```python
from build123d import *

# Parameters (mm, degrees)
F0_R     = 55.8806252639
F1_DEPTH = 12.7


with BuildPart() as f1:
    # F0 (on Top) → F1 (new body)
    with BuildSketch(Plane.XY):
        Circle(F0_R)
        with BuildLine():
            add(Edge.make_bspline(
                [(-8.8274130972, -11.1133217732), (-11.8591704488, -9.6938284468), (-14.8909278004, -9.6938284468)],
                knots=[0, 0, 0, 1, 1, 1], degree=2))
            add(Edge.make_bspline(
                [(-14.8909278004, -9.6938284468), (-19.2896046515, -9.6938284468), (-21.8365144883, -12.6233589127)],
                knots=[0, 0, 0, 1, 1, 1], degree=2))
            add(Edge.make_bspline(
                [(-21.8365144883, -12.6233589127), (-24.3834243251, -15.5528893786), (-24.3834243251, -20.6467090522)],
                knots=[0, 0, 0, 1, 1, 1], degree=2))
            add(Edge.make_bspline(
                [(-24.3834243251, -20.6467090522), (-24.3834243251, -25.8807255975), (-21.9270583013, -28.7401576276)],
                knots=[0, 0, 0, 1, 1, 1], degree=2))
            add(Edge.make_bspline(
                [(-21.9270583013, -28.7401576276), (-19.4706922775, -31.5995896577), (-14.9259770183, -31.5995896577)],
                knots=[0, 0, 0, 1, 1, 1], degree=2))
            add(Edge.make_bspline(
                [(-14.9259770183, -31.5995896577), (-12.133722656, -31.5995896577), (-8.55286089, -30.5948454101)],
                knots=[0, 0, 0, 1, 1, 1], degree=2))
            Line((-8.55286089, -30.5948454101), (-8.55286089, -33.3111598003))
            add(Edge.make_bspline(
                [(-8.55286089, -33.3111598003), (-11.3275906434, -34.3567948021), (-15.3991414605, -34.3567948021)],
                knots=[0, 0, 0, 1, 1, 1], degree=2))
            add(Edge.make_bspline(
                [(-15.3991414605, -34.3567948021), (-21.2932516103, -34.3567948021), (-24.4973342834, -30.7759330361)],
                knots=[0, 0, 0, 1, 1, 1], degree=2))
            add(Edge.make_bspline(
                [(-24.4973342834, -30.7759330361), (-27.7014169565, -27.1950712702), (-27.7014169565, -20.605818298)],
                knots=[0, 0, 0, 1, 1, 1], degree=2))
            add(Edge.make_bspline(
                [(-27.7014169565, -20.605818298), (-27.7014169565, -16.481693654), (-26.1592513673, -13.3798378665)],
                knots=[0, 0, 0, 1, 1, 1], degree=2))
            add(Edge.make_bspline(
                [(-26.1592513673, -13.3798378665), (-24.617085778, -10.2779820791), (-21.705079921, -8.5985403862)],
                knots=[0, 0, 0, 1, 1, 1], degree=2))
            add(Edge.make_bspline(
                [(-21.705079921, -8.5985403862), (-18.7930740641, -6.9190986934), (-14.8500370461, -6.9190986934)],
                knots=[0, 0, 0, 1, 1, 1], degree=2))
            add(Edge.make_bspline(
                [(-14.8500370461, -6.9190986934), (-10.6558139663, -6.9190986934), (-7.5130674245, -8.44958121)],
                knots=[0, 0, 0, 1, 1, 1], degree=2))
            Line((-7.5130674245, -8.44958121), (-8.8274130972, -11.1133217732))
        make_face(mode=Mode.SUBTRACT)
        Polygon((-2.8433452334, 4.6599686343), (2.6139786014, 4.792393521), (5.4573238349, 0.1324248867), (2.8433452334, -4.6599686343), (-2.6139786014, -4.792393521), (-5.4573238349, -0.1324248867), align=None, mode=Mode.SUBTRACT)
        with BuildLine():
            add(Edge.make_bspline(
                [(13.118225471, -17.7074033137), (15.3172801058, -17.2663672866), (17.5040837399, -17.2663672866)],
                knots=[0, 0, 0, 1, 1, 1], degree=2))
            add(Edge.make_bspline(
                [(17.5040837399, -17.2663672866), (21.926695011, -17.2663672866), (24.4626521665, -19.4592964211)],
                knots=[0, 0, 0, 1, 1, 1], degree=2))
            add(Edge.make_bspline(
                [(24.4626521665, -19.4592964211), (26.998609322, -21.6522255555), (26.998609322, -25.4622867892)],
                knots=[0, 0, 0, 1, 1, 1], degree=2))
            add(Edge.make_bspline(
                [(26.998609322, -25.4622867892), (26.998609322, -29.8052665554), (24.2329459024, -32.276905957)],
                knots=[0, 0, 0, 1, 1, 1], degree=2))
            add(Edge.make_bspline(
                [(24.2329459024, -32.276905957), (21.4672824829, -34.7485453585), (16.6036351847, -34.7485453585)],
                knots=[0, 0, 0, 1, 1, 1], degree=2))
            add(Edge.make_bspline(
                [(16.6036351847, -34.7485453585), (11.8747488947, -34.7485453585), (9.3877957422, -33.2355467658)],
                knots=[0, 0, 0, 1, 1, 1], degree=2))
            Line((9.3877957422, -33.2355467658), (9.3877957422, -30.172796578))
            add(Edge.make_bspline(
                [(9.3877957422, -30.172796578), (10.7231548241, -31.0303666306), (12.7139424462, -31.5204066606)],
                knots=[0, 0, 0, 1, 1, 1], degree=2))
            add(Edge.make_bspline(
                [(12.7139424462, -31.5204066606), (14.7047300682, -32.0104466906), (16.6403881869, -32.0104466906)],
                knots=[0, 0, 0, 1, 1, 1], degree=2))
            add(Edge.make_bspline(
                [(16.6403881869, -32.0104466906), (20.0094133935, -32.0104466906), (21.8746282578, -30.4208793432)],
                knots=[0, 0, 0, 1, 1, 1], degree=2))
            add(Edge.make_bspline(
                [(21.8746282578, -30.4208793432), (23.7398431222, -28.8313119957), (23.7398431222, -25.8236913113)],
                knots=[0, 0, 0, 1, 1, 1], degree=2))
            add(Edge.make_bspline(
                [(23.7398431222, -25.8236913113), (23.7398431222, -19.9677129523), (16.5668821824, -19.9677129523)],
                knots=[0, 0, 0, 1, 1, 1], degree=2))
            add(Edge.make_bspline(
                [(16.5668821824, -19.9677129523), (14.7476085709, -19.9677129523), (11.7032348842, -20.5251334864)],
                knots=[0, 0, 0, 1, 1, 1], degree=2))
            Line((11.7032348842, -20.5251334864), (10.0554752832, -19.4715474218))
            Line((10.0554752832, -19.4715474218), (11.1090613478, -6.3752276189))
            Line((11.1090613478, -6.3752276189), (25.0261982011, -6.3752276189))
            Line((25.0261982011, -6.3752276189), (25.0261982011, -9.3032167984))
            Line((25.0261982011, -9.3032167984), (13.8287835145, -9.3032167984))
            Line((13.8287835145, -9.3032167984), (13.118225471, -17.7074033137))
        make_face(mode=Mode.SUBTRACT)
        Polygon((-8.8821777954, 5.6402049959), (-11.8495973103, 5.6402049959), (-14.9195276811, 13.4795878234), (-24.7983370116, 13.4795878234), (-27.830500225, 5.6402049959), (-30.7331760414, 5.6402049959), (-20.9892494161, 30.3938790583), (-18.5775466468, 30.3938790583), align=None, mode=Mode.SUBTRACT)
        with BuildLine():
            Line((18.6679722386, 13.2637759067), (24.385376429, 29.3535589635))
            Line((24.385376429, 29.3535589635), (27.5124241231, 29.3535589635))
            Line((27.5124241231, 29.3535589635), (18.4982025739, 4.3317009695))
            Line((18.4982025739, 4.3317009695), (15.6230711564, 4.3317009695))
            Line((15.6230711564, 4.3317009695), (6.6526611336, 29.3535589635))
            Line((6.6526611336, 29.3535589635), (9.7358973013, 29.3535589635))
            Line((9.7358973013, 29.3535589635), (15.4861601365, 13.1651999724))
            add(Edge.make_bspline(
                [(15.4861601365, 13.1651999724), (16.4773959204, 10.3722151668), (17.0578986448, 7.7380471442)],
                knots=[0, 0, 0, 1, 1, 1], degree=2))
            add(Edge.make_bspline(
                [(17.0578986448, 7.7380471442), (17.6767364546, 10.5091261867), (18.6679722386, 13.2637759067)],
                knots=[0, 0, 0, 1, 1, 1], degree=2))
        make_face(mode=Mode.SUBTRACT)
    extrude(amount=F1_DEPTH)


solid = f1.part
```
Geometry: final body of the model. Coordinates: model frame, mm. Round coordinates to 2 decimals unless told otherwise and drop trailing zeros. Order: outer loops, then holes, each group sorted by start corner. A loop starts at its lowest first (then second) coordinate and runs counter-clockwise, first axis right, second up. Notation, with made-up numbers: (-4.75, -30.5) -> (54.25, -30.5) arc R16 cw to (54.25, -3.5) -> close; hole circle Ø4 at (37, -6.75). An arc over 180 degrees is marked (long way). Use one line per item in the form item = value. Start each with the question number.
1. Pin query (flat end, axial travel): pin 1 Ø6.5 at (x, z) = (17, 9) entering from -Y; pin 2 Ø2.5 at (x, z) = (7.5, 7) entering from -Y; pin 3 Ø3 at (y, z) = (-32, 3) entering from -X. Return the tip coordinate at first contact, or that it passes through.
2. Cut plane C-C (y = 16). Return the cut outline in (x, z), then the cut area to 3 significant figures.
3. Cut plane D-D (x = -13.5). Count the separate pieces of the cut face and the enclosed holes in it, then the cut area to 3 significant figures.
4. Draft query along X for faces 1 (the face through (-44.345, -34.002, 6.261)), 2 (the face through (9.388, -32, 6)), 3 (the face through (12, 1, 0)). Return one class per face: pulls with the +X half, pulls with the -X half, needs draft (parallel to the pull), parting line crosses it, or undercut.
5. Cut plane A-A (y = 2.5). Return the cut outline in (x, z), then the cut area to 3 significant figures.
6. Line query: probe 1 along X at (y, z) = (19, 3.25); probe 2 along X at (y, z) = (11, 8); probe 3 along X at (y, z) = (-32.5, 3.75). Output: solid intervals per line, ascending.
7. Cut plane B-B (x = 0). Return the cut outline in (y, z), then the cut area to 3 significant figures.
Solution:
q1.pin_1 = -54.16
q1.pin_2 = -55.53
q1.pin_3 = -46.82
q2.outline = (-53.54, 0) -> (-26.66, 0) -> (-26.66, 12.7) -> (-53.54, 12.7) -> close; (-12.94, 0) -> (11.44, 0) -> (11.44, 12.7) -> (-12.94, 12.7) -> close; (14.48, 0) -> (19.64, 0) -> (19.64, 12.7) -> (14.48, 12.7) -> close; (22.7, 0) -> (53.54, 0) -> (53.54, 12.7) -> (22.7, 12.7) -> close
q2.area = 1,110 mm^2
q3.separate_pieces = 4
q3.enclosed_holes = 0
q3.area = 1,210 mm^2
q4.face_1 = parting line crosses it
q4.face_2 = undercut
q4.face_3 = needs draft
q5.outline = (-55.82, 0) -> (-4.02, 0) -> (-4.02, 12.7) -> (-55.82, 12.7) -> close; (4.01, 0) -> (55.82, 0) -> (55.82, 12.7) -> (4.01, 12.7) -> close
q5.area = 1,320 mm^2
q6.probe_1 = -52.55 to -25.47, -14.11 to 10.36, 13.41 to 20.71, 23.78 to 52.55
q6.probe_2 = -54.79 to -28.62, -25.76 to -13.95, -10.98 to 13.23, 16.2 to 17.92, 20.9 to 54.79
q6.probe_3 = -45.46 to -22.49, -8.55 to 9.39, 23.97 to 45.46
q7.outline = (-55.88, 0) -> (-4.73, 0) -> (-4.73, 12.7) -> (-55.88, 12.7) -> close; (4.73, 0) -> (55.88, 0) -> (55.88, 12.7) -> (4.73, 12.7) -> close
q7.area = 1,300 mm^2
